Geometry: see drawing. Coordinates: mm, zero at the bounding-box minimum. A direction names the side the tool comes from. Coordinates: 2 decimals unless noted, no trailing zeros. Loops run counter-clockwise (first coordinate to the right, second up) from the corner with the lowest first, then second, coordinate; pieces in that order, holes last.
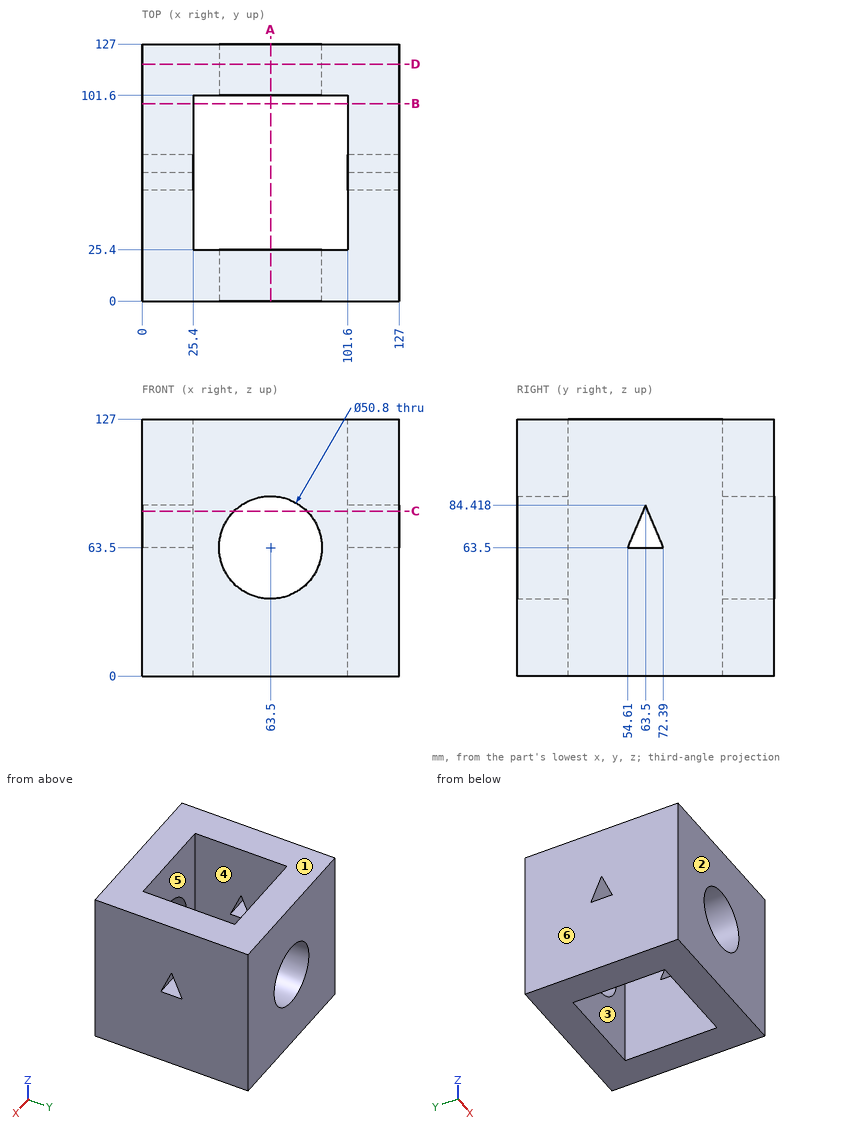
Item 1: Section query B-B (y = 97.5). Output: boundary loops of the cut face in (x, z), then the cut area to 3 significant figures.
Result:
outline: (0, 0) - (25.4, 0) - (25.4, 127) - (0, 127) - close; (101.6, 0) - (127, 0) - (127, 127) - (101.6, 127) - close
area: 6,450 mm2
Item 2: Reachability of the marked faces 5 and 6 from +Z, -Z, +X, -X, +Y, -Y: full face, straight path, thin tool, end or side. Return the list, or none.
Result:
face 5: +Z, -Z
face 6: +Z, -Z, -X, +Y, -Y
Item 3: Section query C-C (z = 81.5). Output: boundary loops of the cut face in (x, y).
Result:
outline: (0, 0) - (45.58, 0) - (45.58, 25.4) - (25.4, 25.4) - (25.4, 62.26) - (0, 62.26) - close; (0, 64.74) - (25.4, 64.74) - (25.4, 101.6) - (45.58, 101.6) - (45.58, 127) - (0, 127) - close; (81.42, 0) - (127, 0) - (127, 62.26) - (101.6, 62.26) - (101.6, 25.4) - (81.42, 25.4) - close; (81.42, 101.6) - (101.6, 101.6) - (101.6, 64.74) - (127, 64.74) - (127, 127) - (81.42, 127) - close
Item 4: Mould query, pull axis Y, two halves, no side actions, for the marked faces 1, 2, 3 and 4. Classes: +Y half, -Y half, draft (parallel to the pull), parting line (faces both ways), or undercut.
Result:
face 1: draft
face 2: -Y half
face 3: undercut
face 4: undercut
Item 5: Section query A-A (x = 63.5). Output: boundary loops of the cut face in (y, z).
Result:
outline: (0, 0) - (25.4, 0) - (25.4, 38.1) - (0, 38.1) - close; (0, 88.9) - (25.4, 88.9) - (25.4, 127) - (0, 127) - close; (101.6, 0) - (127, 0) - (127, 38.1) - (101.6, 38.1) - close; (101.6, 88.9) - (127, 88.9) - (127, 127) - (101.6, 127) - close
Item 6: Contact query for flat-ended pins moving along their axis: P1, Ø5, axis at x = 16, z = 57, coming from the -Y side; P2, Ø12, axis at x = 68.5, y = 91, coming from the -Z side. Output: stop coordinate, or through.
Result:
P1: stops at y = 0
P2: passes through
Item 7: Line query: L1, parallel to X at y = 49.5, z = 69; L2, parallel to Z at x = 63.5, y = 19. Output: solid intervals per line, ascending.
Result:
L1: x = 0 to 25.4, 101.6 to 127
L2: z = 0 to 38.1, 88.9 to 127
Item 8: Section query D-D (y = 117). Output: boundary loops of the cut face in (x, z).
Result:
outline: (0, 0) - (127, 0) - (127, 127) - (0, 127) - close; hole circle Ø50.8 at (63.5, 63.5)
